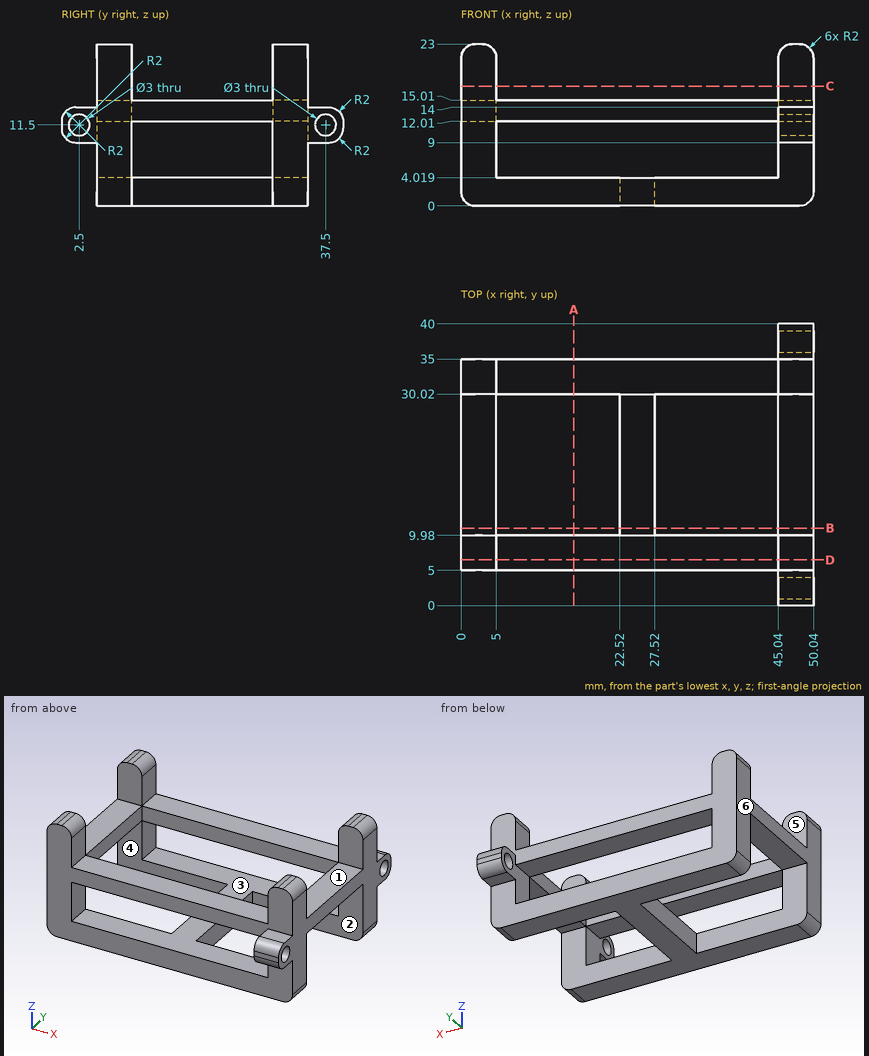
Job drawing, mm, ordinate dimensions from the low corner. One solid piece. A direction names the side the tool comes from. Coordinates: 2 decimals unless noted, no trailing zeros. Loops run counter-clockwise (first coordinate to the right, second up) from the corner with the lowest first, then second, coordinate; pieces in that order, holes last. Notation, with made-up numbers: (45.5, 59) - (59.5, 59) arc R24 cw to (59.5, 93) - close; hole circle Ø6 at (34.25, 71). An arc over 180 degrees is marked (long way). Answer as a JSON object with one key per item and string values. Group by question number.
(1) Tool access for the marked faces 1, 2 and 3: list every direction of +Z, -Z, +X, -X, +Y, -Y with a clear straight run to the whole face (end or side of a thin tool).
(2) Probe line 1 along Y through (x, z) = (48.6, 11.5); line 2 along Y through (x, z) = (45.5, 10.25) (1 decimal); line 3 along X through (y, z) = (14.5, 13.25). List the from-to ranges inside material, lowest first.
(3) Flat gauge pins, fed straight in: pin 1 (4 mm diameter, centred on x = 21, z = 15.5, fed in from -Y); pin 2 (5 mm diameter, centred on x = 26.5, y = 20.5, fed in from -Z); pin 3 (4 mm diameter, centred on x = 24, z = 3, fed in from +Y); pin 4 (5.5 mm diameter, centred on x = 46.5, y = 23.5, fed in from +Z). Where does each tip first touch, or does it go through?
(4) Two-plate mould, pull along Y, no slides. Class the marked faces 4, 5 and 6: released by +Y, released by -Y, zero draft, split by the parting line, or undercut.
(5) Cut at C-C (z = 17). Give the cut face in (x, y).
(6) Cut at D-D (y = 6.5). Give the cut face in (x, z), then the cut area to 3 significant figures.
(7) Cut at A-A (x = 16). Give the cut face in (y, z).
(8) Cut at B-B (y = 11). Give the cut face in (x, z).
Geometry says:
{
 "1": {"face 1": "+Z, +X, -X", "face 2": "-Z, +X", "face 3": "+Y, -Y"},
 "2": {"line 1": "y = 0 to 1, 4 to 9.98, 30.02 to 36, 39 to 40", "line 2": "y = 0.1 to 1.7, 3.3 to 10, 30 to 36.7, 38.3 to 39.9", "line 3": "x = 0 to 5, 45.04 to 50.04"},
 "3": {"pin 1": "stops at y = 5", "pin 2": "stops at z = 0", "pin 3": "stops at y = 35", "pin 4": "stops at z = 15.01"},
 "4": {"face 4": "undercut", "face 5": "undercut", "face 6": "zero draft"},
 "5": {"outline": "(0, 5) - (5, 5) - (5, 9.98) - (0, 9.98) - close; (0, 30.02) - (5, 30.02) - (5, 35) - (0, 35) - close; (45.04, 5) - (50.04, 5) - (50.04, 9.98) - (45.04, 9.98) - close; (45.04, 30.02) - (50.04, 30.02) - (50.04, 35) - (45.04, 35) - close"},
 "6": {"outline": "(0, 2) arc R2 ccw to (2, 0) - (48.04, 0) arc R2 ccw to (50.04, 2) - (50.04, 21) arc R2 ccw to (48.04, 23) - (47.04, 23) arc R2 ccw to (45.04, 21) - (45.04, 15.01) - (5, 15.01) - (5, 21) arc R2 ccw to (3, 23) - (2, 23) arc R2 ccw to (0, 21) - close; hole (5, 4.02) - (45.04, 4.02) - (45.04, 12.01) - (5, 12.01) - close", "area": "506 mm^2"},
 "7": {"outline": "(5, 0) - (9.98, 0) - (9.98, 4.02) - (5, 4.02) - close; (5, 12.01) - (9.98, 12.01) - (9.98, 15.01) - (5, 15.01) - close; (30.02, 0) - (35, 0) - (35, 4.02) - (30.02, 4.02) - close; (30.02, 12.01) - (35, 12.01) - (35, 15.01) - (30.02, 15.01) - close"},
 "8": {"outline": "(0, 12.01) - (5, 12.01) - (5, 15.01) - (0, 15.01) - close; (22.52, 0) - (27.52, 0) - (27.52, 4.02) - (22.52, 4.02) - close; (45.04, 12.01) - (50.04, 12.01) - (50.04, 15.01) - (45.04, 15.01) - close"}
}
